The figure shows three views and two pictorial views of one solid part (mm, origin at its lowest corner). Answer the questions. Coordinates: 2 decimals unless noted, no trailing zeros. Write each loop counter-clockwise with the first axis right and the second up, starting at its lowest first coordinate (ties: lowest second). Pieces come first, ordered by that corner, then holes.
Item 1: Straight lines are drawn through the part: probe 1 along X at (y, z) = (0.95, 10); probe 2 along X at (y, z) = (2.25, 74.15); probe 3 along Z at (x, y) = (10.5, 0.35). For each, find the intervals that lie inside material, in ascending order.
Item 2: Section B-B (x = 46.85) is taken. Give the vertices of the cut face in (y, z), then the cut area to 3 significant figures.
Item 3: This flat-tipped pin is pushed along its axis until it touches: P1, Ø6, axis at x = 135.5, z = 76, coming from the -Y side. Where does it stop, or does it pass through?
Item 4: Section C-C (y = 1.8) is taken. State how many separate pieces and enclosed holes the cut face has, then the cut area to 3 significant figures.
Item 5: Section A-A (z = 15.85) is taken. Give the vertices of the cut face in (x, y).
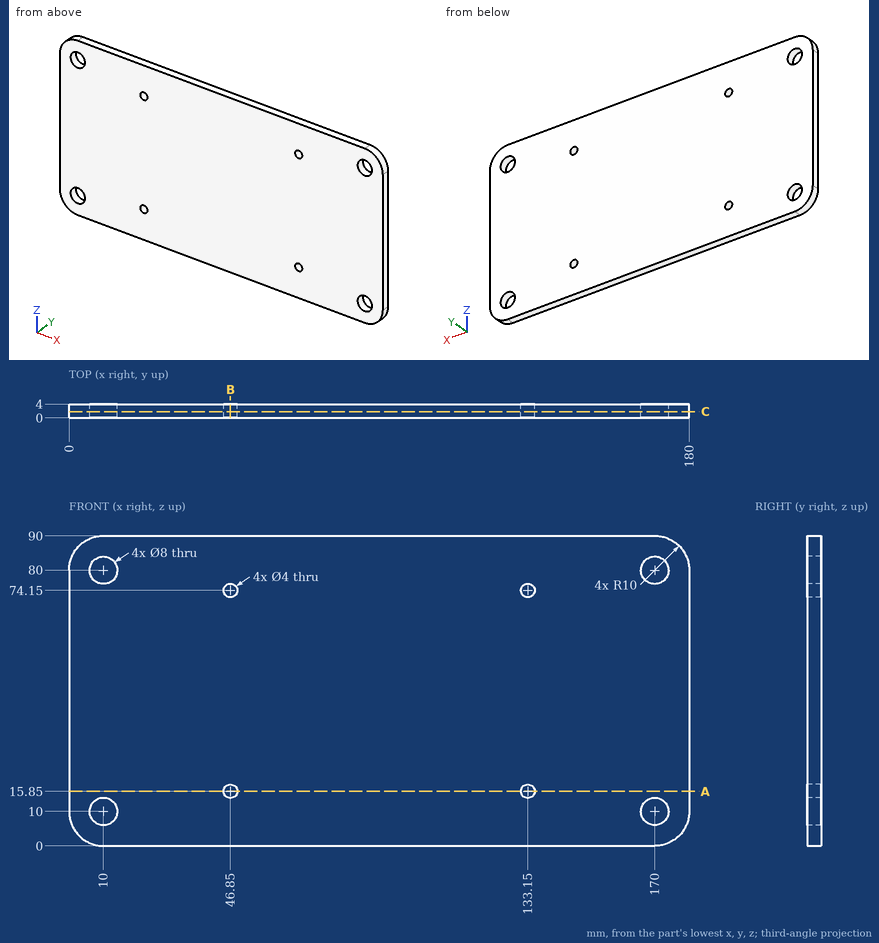
Established:
1. probe 1: x = 0 to 6, 14 to 166, 174 to 180
1. probe 2: x = 0 to 44.85, 48.85 to 131.15, 135.15 to 180
1. probe 3: z = 0 to 6.03, 13.97 to 76.03, 83.97 to 90
2. outline: (0, 0) - (4, 0) - (4, 13.85) - (0, 13.85) - close; (0, 17.85) - (4, 17.85) - (4, 72.15) - (0, 72.15) - close; (0, 76.15) - (4, 76.15) - (4, 90) - (0, 90) - close
2. area: 328 mm2
3. P1: stops at y = 0
4. separate pieces: 1
4. enclosed holes: 8
4. area: 15,900 mm2
5. outline: (0, 0) - (44.85, 0) - (44.85, 4) - (0, 4) - close; (48.85, 0) - (131.15, 0) - (131.15, 4) - (48.85, 4) - close; (135.15, 0) - (180, 0) - (180, 4) - (135.15, 4) - close
